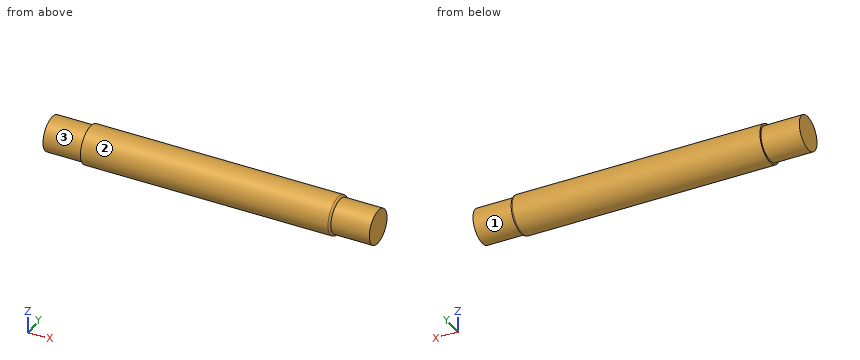
from build123d import *

# Parameters (mm, degrees)
FILLET_1_R = 2


with BuildPart() as part:
    # 草图8 → 旋转1 (revolve)
    with BuildSketch(Plane.XY, mode=Mode.PRIVATE) as revolve_1_sk:
        Polygon((0, 0), (340, 0), (340, 18), (300, 18), (300, 20), (40, 20), (40, 18), (0, 18), align=None)
    revolve(revolve_1_sk.sketch.rotate(Axis((0, 0, 0), (1, 0, 0)), 90), axis=Axis((0, 0, 0), (1, 0, 0)))

    # 圆角1
    fillet_1_edges = [part.edges().sort_by_distance(p)[0] for p in [
        (300, 0, -20),
    ]]
    fillet(fillet_1_edges, radius=FILLET_1_R - 0.0001)  # a hair under: the kernel refuses the full size


solid = part.part
The model under review builds one solid part; all positions refer to its coordinate system, in mm. Face numbers are marked on the shaded views. A direction names the side the tool comes from. Give positions to 0.01 mm unless a question says otherwise; leave off trailing zeros. Write each loop counter-clockwise with the first axis right and the second up, starting at its lowest first coordinate (ties: lowest second). Pieces come first, ordered by that corner, then holes. Notation, with made-up numbers: M -9,48 L 18,48 A35 cw 18,81 Z; hole C -3.5,87 d3. An arc over 180 degrees is marked long. One line per question, with ' | ' between items. Start each with the question number.
Item 1: For the marked faces 1, 2 and 3, list the 3-axis set-ups (+Z, -Z, +X, -X, +Y, -Y) from which the entire face can be reached by the end or side of a thin tool; tool diameter is ignored.
Item 2: We need section C-C on x = 211.5. Write out the cut boundary in (y, z), plus the area to 3 significant figures.
Item 3: For pin 1 (12 mm diameter, centred on x = 280.5, y = 7.5, fed in from -Z); pin 2 (1.5 mm diameter, centred on x = 225.5, z = 8, fed in from +Y); pin 3 (2 mm diameter, centred on x = 48.5, y = 12, fed in from +Z), all flat-tipped, find the tip position at first contact; note any pin that passes through.
Item 4: Wall thickness on line 1 (X direction, y = -16.5, z = 7.5); line 2 (Y direction, x = 312, z = -1); line 3 (Y direction, x = 186, z = -14): over which ranges is each line inside the solid? List them lowest first. Write a range as from..to.
Results found:
1) face 1: +X | face 2: +X, -X | face 3: -X
2) outline: C 0,0 d40 | area: 1,260 mm2
3) pin 1: stops at z = -19.94 | pin 2: stops at y = 18.64 | pin 3: stops at z = 16.7
4) line 1: x = 40..300 | line 2: y = -17.97..17.97 | line 3: y = -14.28..14.28
